For this review, take the finished solid that the model builds, in its own axes (mm). Round coordinates to 2 decimals unless told otherwise and drop trailing zeros. Loops run counter-clockwise (first coordinate to the right, second up) from the corner with the lowest first, then second, coordinate; pieces in that order, holes last. Notation, with made-up numbers: (-30.75, -30.75) -> (-6.75, -30.75) arc R23 cw to (-6.75, -9.75) -> close; hole circle Ø10 at (-38, -28). An arc over 180 degrees is marked (long way). Write each question's results on one line, items separated by ' | '.
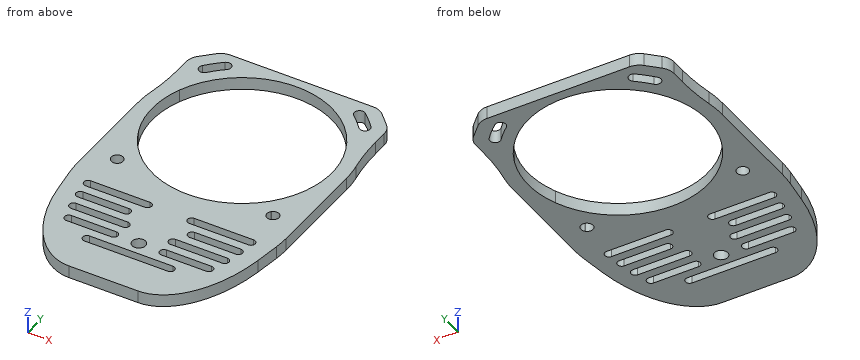
```python
from build123d import *

# Parameters (mm, degrees)
SKETCH1_R           = 1.6
SKETCH1_R_2         = 1.25
SKETCH1_R_3         = 4
BOSS_EXTRUDE1_DEPTH = 3
SKETCH2_R           = 21.5
CUT_EXTRUDE1_DEPTH  = 4.0000001


with BuildPart() as part:
    # Sketch1 → Boss-Extrude1 (new body)
    with BuildSketch(Plane.XY):
        with BuildLine():
            Line((-8.26270655, -49), (8.26270655, -49))
            add(Edge.make_bspline(
                [(8.26270655, -49), (20.894736842, -49), (23.936908844, -27.324524486)],
                knots=[0.034552975, 0.034552975, 0.034552975, 1.433171116, 1.433171116, 1.433171116], degree=2, weights=[1, 0.765287114, 1]))
            Line((23.936908844, -27.324524486), (24.760179539, -21.458720786))
            add(Edge.make_bspline(
                [(24.760179539, -21.458720786), (25, -19.75), (25, -18.013516259)],
                knots=[1.391738704, 1.391738704, 1.391738704, 1.570796327, 1.570796327, 1.570796327], degree=2, weights=[1, 0.995994972, 1]))
            Line((25, -18.013516259), (25, 6))
            ThreePointArc((25, 6), (24.89561541, 8.282177323), (24.583333333, 10.545296714))
            ThreePointArc((24.583333333, 10.545296714), (23.958769179, 15.071535497), (23.75, 19.635890143))
            Line((23.75, 19.635890143), (23.75, 23.093145751))
            ThreePointArc((23.75, 23.093145751), (23.44551813, 24.62387948), (22.578427125, 25.921572875))
            Line((22.578427125, 25.921572875), (19.921572875, 28.578427125))
            ThreePointArc((19.921572875, 28.578427125), (18.62387948, 29.44551813), (17.093145751, 29.75))
            Line((17.093145751, 29.75), (-17.093145751, 29.75))
            ThreePointArc((-17.093145751, 29.75), (-18.62387948, 29.44551813), (-19.921572875, 28.578427125))
            Line((-19.921572875, 28.578427125), (-22.578427125, 25.921572875))
            ThreePointArc((-22.578427125, 25.921572875), (-23.44551813, 24.62387948), (-23.75, 23.093145751))
            Line((-23.75, 23.093145751), (-23.75, 19.635890143))
            ThreePointArc((-23.75, 19.635890143), (-23.958769179, 15.071535497), (-24.583333333, 10.545296714))
            ThreePointArc((-24.583333333, 10.545296714), (-24.89561541, 8.282177323), (-25, 6))
            Line((-25, 6), (-25, -18.013516259))
            add(Edge.make_bspline(
                [(-25, -18.013516259), (-25, -19.75), (-24.760179539, -21.458720786)],
                knots=[4.71238898, 4.71238898, 4.71238898, 4.891446603, 4.891446603, 4.891446603], degree=2, weights=[1, 0.995994972, 1]))
            Line((-24.760179539, -21.458720786), (-23.936908844, -27.324524486))
            add(Edge.make_bspline(
                [(-23.936908844, -27.324524486), (-20.894736842, -49), (-8.26270655, -49)],
                knots=[4.850014191, 4.850014191, 4.850014191, 6.248632332, 6.248632332, 6.248632332], degree=2, weights=[1, 0.765287114, 1]))
        make_face()
        with Locations((0, -35)):
            Circle(SKETCH1_R, mode=Mode.SUBTRACT)
        with Locations((-6.257723989, 7.758092853)):
            Circle(SKETCH1_R_2, mode=Mode.SUBTRACT)
        with Locations((6.257723989, 4.241907147)):
            Circle(SKETCH1_R_2, mode=Mode.SUBTRACT)
        with Locations((0, 6)):
            Circle(SKETCH1_R_3, mode=Mode.SUBTRACT)
        with BuildLine():
            Line((5.284461571, -23.8125), (19.521169673, -23.8125))
            ThreePointArc((19.521169673, -23.8125), (20.521169673, -22.8125), (19.521169673, -21.8125))
            Line((19.521169673, -21.8125), (5.284461571, -21.8125))
            ThreePointArc((5.284461571, -21.8125), (4.284461571, -22.8125), (5.284461571, -23.8125))
        make_face(mode=Mode.SUBTRACT)
        with BuildLine():
            Line((-5.690263266, -29.9375), (-18.129953736, -29.9375))
            ThreePointArc((-18.129953736, -29.9375), (-19.129953736, -30.9375), (-18.129953736, -31.9375))
            Line((-18.129953736, -31.9375), (-5.690263266, -31.9375))
            ThreePointArc((-5.690263266, -31.9375), (-4.690263266, -30.9375), (-5.690263266, -29.9375))
        make_face(mode=Mode.SUBTRACT)
        with BuildLine():
            Line((-6, -34), (-16.793141988, -34))
            ThreePointArc((-16.793141988, -34), (-17.793141988, -35), (-16.793141988, -36))
            Line((-16.793141988, -36), (-6, -36))
            ThreePointArc((-6, -36), (-5, -35), (-6, -34))
        make_face(mode=Mode.SUBTRACT)
        with BuildLine():
            Line((-7.838149252, -25.875), (-18.950227736, -25.875))
            ThreePointArc((-18.950227736, -25.875), (-19.950227736, -26.875), (-18.950227736, -27.875))
            Line((-18.950227736, -27.875), (-7.838149252, -27.875))
            ThreePointArc((-7.838149252, -27.875), (-6.838149252, -26.875), (-7.838149252, -25.875))
        make_face(mode=Mode.SUBTRACT)
        with BuildLine():
            Line((-5.284461571, -21.8125), (-19.521169673, -21.8125))
            ThreePointArc((-19.521169673, -21.8125), (-20.521169673, -22.8125), (-19.521169673, -23.8125))
            Line((-19.521169673, -23.8125), (-5.284461571, -23.8125))
            ThreePointArc((-5.284461571, -23.8125), (-4.284461571, -22.8125), (-5.284461571, -21.8125))
        make_face(mode=Mode.SUBTRACT)
        with BuildLine():
            Line((7.838149252, -27.875), (18.950227736, -27.875))
            ThreePointArc((18.950227736, -27.875), (19.950227736, -26.875), (18.950227736, -25.875))
            Line((18.950227736, -25.875), (7.838149252, -25.875))
            ThreePointArc((7.838149252, -25.875), (6.838149252, -26.875), (7.838149252, -27.875))
        make_face(mode=Mode.SUBTRACT)
        with BuildLine():
            Line((6, -36), (16.793141988, -36))
            ThreePointArc((16.793141988, -36), (17.793141988, -35), (16.793141988, -34))
            Line((16.793141988, -34), (6, -34))
            ThreePointArc((6, -34), (5, -35), (6, -36))
        make_face(mode=Mode.SUBTRACT)
        with BuildLine():
            Line((-10, -40.0625), (10, -40.0625))
            ThreePointArc((10, -40.0625), (11, -39.0625), (10, -38.0625))
            Line((10, -38.0625), (-10, -38.0625))
            ThreePointArc((-10, -38.0625), (-11, -39.0625), (-10, -40.0625))
        make_face(mode=Mode.SUBTRACT)
        with BuildLine():
            Line((5.690263266, -31.9375), (18.129953736, -31.9375))
            ThreePointArc((18.129953736, -31.9375), (19.129953736, -30.9375), (18.129953736, -29.9375))
            Line((18.129953736, -29.9375), (5.690263266, -29.9375))
            ThreePointArc((5.690263266, -29.9375), (4.690263266, -30.9375), (5.690263266, -31.9375))
        make_face(mode=Mode.SUBTRACT)
        with BuildLine():
            Line((12.412191587, 10), (17.12454379, 10))
            ThreePointArc((17.12454379, 10), (19.615066366, 11.327487729), (19.901496836, 14.135135135))
            ThreePointArc((19.901496836, 14.135135135), (0, 27.5), (-19.901496836, 14.135135135))
            ThreePointArc((-19.901496836, 14.135135135), (-19.615066366, 11.327487729), (-17.12454379, 10))
            Line((-17.12454379, 10), (-12.412191587, 10))
            ThreePointArc((-12.412191587, 10), (-10.899090902, 10.409531642), (-9.799098622, 11.526315789))
            ThreePointArc((-9.799098622, 11.526315789), (0, 17.25), (9.799098622, 11.526315789))
            ThreePointArc((9.799098622, 11.526315789), (10.899090902, 10.409531642), (12.412191587, 10))
        make_face(mode=Mode.SUBTRACT)
        with BuildLine():
            Line((17.12454379, 2), (12.412191587, 2))
            ThreePointArc((12.412191587, 2), (10.899090902, 1.590468358), (9.799098622, 0.473684211))
            ThreePointArc((9.799098622, 0.473684211), (0, -5.25), (-9.799098622, 0.473684211))
            ThreePointArc((-9.799098622, 0.473684211), (-10.899090902, 1.590468358), (-12.412191587, 2))
            Line((-12.412191587, 2), (-17.12454379, 2))
            ThreePointArc((-17.12454379, 2), (-19.615066366, 0.672512271), (-19.901496836, -2.135135135))
            ThreePointArc((-19.901496836, -2.135135135), (0, -15.5), (19.901496836, -2.135135135))
            ThreePointArc((19.901496836, -2.135135135), (19.615066366, 0.672512271), (17.12454379, 2))
        make_face(mode=Mode.SUBTRACT)
        with BuildLine():
            ThreePointArc((-15.196569313, 25.146541488), (-15.032451192, 26.906673654), (-16.792583358, 27.070791775))
            ThreePointArc((-16.792583358, 27.070791775), (-18.571456346, 25.459260737), (-20.203027197, 23.698750028))
            ThreePointArc((-20.203027197, 23.698750028), (-20.058850519, 21.936872312), (-18.296972803, 22.081048991))
            ThreePointArc((-18.296972803, 22.081048991), (-16.813726575, 23.681513271), (-15.196569313, 25.146541488))
        make_face(mode=Mode.SUBTRACT)
        with BuildLine():
            ThreePointArc((-19.691847489, -13.623229665), (-19.657568517, -13.657568517), (-19.623229665, -13.691847489))
            ThreePointArc((-19.623229665, -13.691847489), (-17.643333693, -13.688391915), (-17.646789267, -11.708495943))
            ThreePointArc((-17.646789267, -11.708495943), (-17.67766953, -11.67766953), (-17.708495943, -11.646789267))
            ThreePointArc((-17.708495943, -11.646789267), (-19.688391915, -11.643333693), (-19.691847489, -13.623229665))
        make_face(mode=Mode.SUBTRACT)
        with BuildLine():
            ThreePointArc((17.646789267, -11.708495943), (17.643333693, -13.688391915), (19.623229665, -13.691847489))
            ThreePointArc((19.623229665, -13.691847489), (19.657568517, -13.657568517), (19.691847489, -13.623229665))
            ThreePointArc((19.691847489, -13.623229665), (19.688391915, -11.643333693), (17.708495943, -11.646789267))
            ThreePointArc((17.708495943, -11.646789267), (17.67766953, -11.67766953), (17.646789267, -11.708495943))
        make_face(mode=Mode.SUBTRACT)
        with BuildLine():
            ThreePointArc((18.296972803, 22.081048991), (20.058850519, 21.936872312), (20.203027197, 23.698750028))
            ThreePointArc((20.203027197, 23.698750028), (18.571456346, 25.459260737), (16.792583358, 27.070791775))
            ThreePointArc((16.792583358, 27.070791775), (15.032451192, 26.906673654), (15.196569313, 25.146541488))
            ThreePointArc((15.196569313, 25.146541488), (16.813726575, 23.681513271), (18.296972803, 22.081048991))
        make_face(mode=Mode.SUBTRACT)
    extrude(amount=BOSS_EXTRUDE1_DEPTH)

    # Sketch2 → Cut-Extrude1 (cut, through all)
    with BuildSketch(Plane.XY.offset(3)):
        with Locations((0, 6)):
            Circle(SKETCH2_R)
    extrude(amount=-CUT_EXTRUDE1_DEPTH, mode=Mode.SUBTRACT)


solid = part.part
```
1. Consider section C-C (y = 2). State the section outline as (x, z) points.
Values found:
outline: (-25, 0) -> (-21.12, 0) -> (-21.12, 3) -> (-25, 3) -> close; (21.12, 0) -> (25, 0) -> (25, 3) -> (21.12, 3) -> close
2. Consider section B-B (z = 1.35). Give the number of separate pieces and of enclosed holes in the cut face, plus the area to 3 significant figures.
Values found:
separate pieces: 1 | enclosed holes: 15 | area: 1,870 mm2
3. Consider section A-A (x = 0). State the section outline as (y, z) points.
Values found:
outline: (-49, 0) -> (-40.06, 0) -> (-40.06, 3) -> (-49, 3) -> close; (-38.06, 0) -> (-36.6, 0) -> (-36.6, 3) -> (-38.06, 3) -> close; (-33.4, 0) -> (-15.5, 0) -> (-15.5, 3) -> (-33.4, 3) -> close; (27.5, 0) -> (29.75, 0) -> (29.75, 3) -> (27.5, 3) -> close
4. To check wall thickness, follow probe 1 along Y at (x, z) = (0, 2.45); probe 2 along Y at (x, z) = (-2, 1.55); probe 3 along Y at (x, z) = (-0.5, 1.15). State the ranges of each line that lie inside material, in increasing order.
Values found:
probe 1: y = -49 to -40.06, -38.06 to -36.6, -33.4 to -15.5, 27.5 to 29.75 | probe 2: y = -49 to -40.06, -38.06 to -15.41, 27.41 to 29.75 | probe 3: y = -49 to -40.06, -38.06 to -36.52, -33.48 to -15.49, 27.49 to 29.75
5. For pin 1 (1.5 mm diameter, centred on x = 15, z = 2, fed in from -Y); pin 2 (1.5 mm diameter, centred on x = -14, z = 2, fed in from -Y); pin 3 (0.9 mm diameter, centred on x = 12, z = 1, fed in from -Y), all flat-tipped, find the tip position at first contact; note any pin that passes through.
Values found:
pin 1: stops at y = -46.9 | pin 2: stops at y = -47.55 | pin 3: stops at y = -48.38
